Work out the finished part from the listing and answer in its coordinate system (mm). A direction names the side the tool comes from. Coordinates: 2 decimals unless noted, no trailing zeros. Write each loop counter-clockwise with the first axis right and the second up, starting at its lowest first coordinate (ties: lowest second). Pieces come first, ordered by that corner, then holes. Notation, with made-up numbers: (7.25, 45.25) - (45.25, 45.25) arc R27 cw to (45.25, 84.25) - close; hole circle Ø6 at (68, 46.5). An arc over 180 degrees is marked (long way). Use a Markdown table: item, result. Add a question column.
(1) A tool of negligible diameter and unlimited length cuts with its end or side. For faces 1 (the face through (35, 20, 1)), 2 (the face through (10, 30, 1)), 3 (the face through (40, 10, 1)), from which of +Z, -Z, +X, -X, +Y, -Y can it reach the whole face along a straight path? Write none if from no direction.
(2) The part is cut by section D-D, the plane y = 24. Give the vertices of the cut face in (x, z) (3 decimals).
(3) Given pin 1 Ø1 at (x, z) = (35.5, 1.5) entering from +Y; pin 2 Ø3 at (x, y) = (14, 36) entering from +Z; pin 3 Ø1.5 at (y, z) = (26, 2) entering from -X; pin 4 Ø0.9 at (y, z) = (33, 1) entering from +X, each flat-ended and moving along its own axis, determine where each tip first touches the part or whether it passes through.
(4) The part is cut by section C-C, the plane z = 2.4. State how many separate pieces and enclosed holes the cut face has, then the cut area to 3 significant figures.
(5) The part is cut by section A-A, the plane y = 4. Give the vertices of the cut face in (x, z) (3 decimals).
(6) The part is cut by section B-B, the plane x = 14. Give the vertices of the cut face in (y, z) (3 decimals), then the cut area to 3 significant figures.
(7) Find the intervals of material crossed by line 1 (Y direction, x = 26, z = 2.1) (3 decimals); line 2 (Y direction, x = 36, z = 0.7) (3 decimals); line 3 (X direction, y = 27, z = 1.6), in increasing order. Write a range as from..to.
(8) For a pull along Y with two mould halves and no side action, classify faces 4 (the face through (5, 20, 1)), 5 (the face through (24.427, 36.069, 1.521)), 6 (the face through (20, 16, 0)) as released by +Y, released by -Y, zero draft, split by the parting line, or undercut.
from build123d import *

# Parameters (mm, degrees)
EXTRUDE_1_DEPTH     = 3
SKETCH_2_R          = 1.575
CUT_EXTRUDE_1_DEPTH = 3


with BuildPart() as part:
    # 草图1 → 凸台-拉伸1 (new body)
    with BuildSketch(Plane.XY):
        Polygon((0, 0), (40, 0), (40, 20), (30, 20), (30, 40), (10, 40), (10, 20), (0, 20), align=None)
    extrude(amount=EXTRUDE_1_DEPTH)

    # 草图2 → 切除-拉伸1 (cut)
    with BuildSketch(Plane.XY.offset(3)):
        with Locations((14, 36)):
            Circle(SKETCH_2_R)
        with Locations((26, 36)):
            Circle(SKETCH_2_R)
        with Locations((26, 24)):
            Circle(SKETCH_2_R)
        with Locations((14, 24)):
            Circle(SKETCH_2_R)
        with Locations((4, 16)):
            Circle(SKETCH_2_R)
        with Locations((4, 4)):
            Circle(SKETCH_2_R)
        with Locations((14, 16)):
            Circle(SKETCH_2_R)
        with Locations((14, 4)):
            Circle(SKETCH_2_R)
        with Locations((36, 16)):
            Circle(SKETCH_2_R)
        with Locations((36, 4)):
            Circle(SKETCH_2_R)
        with Locations((26, 4)):
            Circle(SKETCH_2_R)
        with Locations((26, 16)):
            Circle(SKETCH_2_R)
    extrude(amount=-CUT_EXTRUDE_1_DEPTH, mode=Mode.SUBTRACT)


solid = part.part
Model answer:
| question | item | result |
|---|---|---|
| 1 | face 1 | +Z, -Z, +X, +Y |
| 1 | face 2 | +Z, -Z, -X, +Y |
| 1 | face 3 | +Z, -Z, +X, +Y, -Y |
| 2 | outline | (10, 0) - (12.425, 0) - (12.425, 3) - (10, 3) - close; (15.575, 0) - (24.425, 0) - (24.425, 3) - (15.575, 3) - close; (27.575, 0) - (30, 0) - (30, 3) - (27.575, 3) - close |
| 3 | pin 1 | y = 20 |
| 3 | pin 2 | through |
| 3 | pin 3 | x = 10 |
| 3 | pin 4 | x = 30 |
| 4 | separate pieces | 1 |
| 4 | enclosed holes | 12 |
| 4 | area | 1,110 mm^2 |
| 5 | outline | (0, 0) - (2.425, 0) - (2.425, 3) - (0, 3) - close; (5.575, 0) - (12.425, 0) - (12.425, 3) - (5.575, 3) - close; (15.575, 0) - (24.425, 0) - (24.425, 3) - (15.575, 3) - close; (27.575, 0) - (34.425, 0) - (34.425, 3) - (27.575, 3) - close; (37.575, 0) - (40, 0) - (40, 3) - (37.575, 3) - close |
| 6 | outline | (0, 0) - (2.425, 0) - (2.425, 3) - (0, 3) - close; (5.575, 0) - (14.425, 0) - (14.425, 3) - (5.575, 3) - close; (17.575, 0) - (22.425, 0) - (22.425, 3) - (17.575, 3) - close; (25.575, 0) - (34.425, 0) - (34.425, 3) - (25.575, 3) - close; (37.575, 0) - (40, 0) - (40, 3) - (37.575, 3) - close |
| 6 | area | 82.2 mm^2 |
| 7 | line 1 | 0..2.425, 5.575..14.425, 17.575..22.425, 25.575..34.425, 37.575..40 |
| 7 | line 2 | 0..2.425, 5.575..14.425, 17.575..20 |
| 7 | line 3 | 10..30 |
| 8 | face 4 | released by +Y |
| 8 | face 5 | undercut |
| 8 | face 6 | zero draft |
